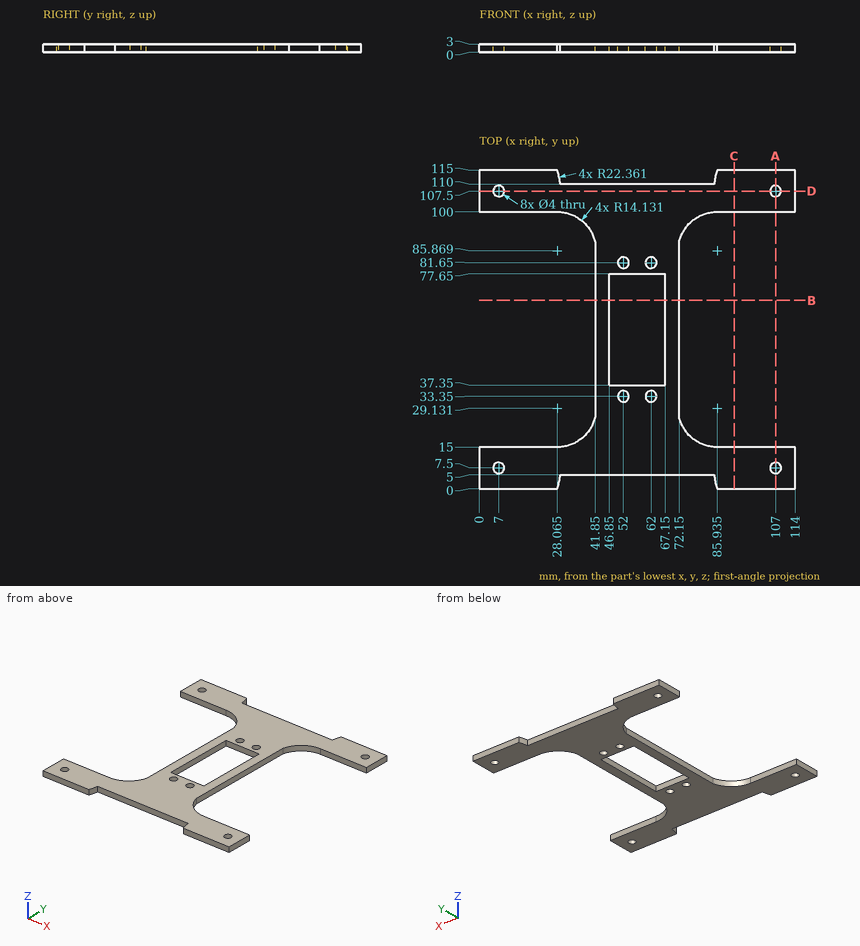
Verification items for this drawing (mm, ordinates from the low corner). Give positions to 0.01 mm unless a question says otherwise; leave off trailing zeros. Loops run counter-clockwise (first coordinate to the right, second up) from the corner with the lowest first, then second, coordinate; pieces in that order, holes last.
(1) Section check C-C on x = 92. Record the cut outline in (y, z).
From the geometry:
outline: (0, 0) - (15, 0) - (15, 3) - (0, 3) - close; (100, 0) - (115, 0) - (115, 3) - (100, 3) - close
(2) Section check A-A on x = 107. Record the cut outline in (y, z).
From the geometry:
outline: (0, 0) - (5.5, 0) - (5.5, 3) - (0, 3) - close; (9.5, 0) - (15, 0) - (15, 3) - (9.5, 3) - close; (100, 0) - (105.5, 0) - (105.5, 3) - (100, 3) - close; (109.5, 0) - (115, 0) - (115, 3) - (109.5, 3) - close
(3) Section check B-B on y = 68. Record the cut outline in (x, z), then the cut area to 3 significant figures.
From the geometry:
outline: (41.85, 0) - (46.85, 0) - (46.85, 3) - (41.85, 3) - close; (67.15, 0) - (72.15, 0) - (72.15, 3) - (67.15, 3) - close
area: 30.0 mm2
(4) Depth check by flat-ended pin: pin 1 Ø6.5 at (x, y) = (7, 7.5) entering from -Z; pin 2 Ø0.9 at (y, z) = (57, 1.5) entering from +X; pin 3 Ø3 at (x, y) = (107, 107.5) entering from +Z. Enter the tip coordinate at first touch or a pass-through.
From the geometry:
pin 1: stops at z = 0
pin 2: stops at x = 72.15
pin 3: passes through
(5) Section check D-D on y = 107.5. Record the cut outline in (x, z), then the cut area to 3 significant figures.
From the geometry:
outline: (0, 0) - (5, 0) - (5, 3) - (0, 3) - close; (9, 0) - (105, 0) - (105, 3) - (9, 3) - close; (109, 0) - (114, 0) - (114, 3) - (109, 3) - close
area: 318 mm2
(6) Thickness scan on L1, parallel to Y at x = 107, z = 1.4; L2, parallel to Y at x = 52, z = 0.95; L3, parallel to X at y = 107.5, z = 1.8. Record the ranges inside material, lowest first.
From the geometry:
L1: y = 0 to 5.5, 9.5 to 15, 100 to 105.5, 109.5 to 115
L2: y = 5 to 31.35, 35.35 to 37.35, 77.65 to 79.65, 83.65 to 110
L3: x = 0 to 5, 9 to 105, 109 to 114
